```python
from build123d import *

# Parameters (mm, degrees)
F0_W     = 760
F0_H     = 80
F1_DEPTH = 50
F2_W     = 45
F2_H     = 65
F2_W_2   = 50
F2_W_3   = 55
F3_DEPTH = 50


with BuildPart() as f1:
    # F0 (on Front) → F1 (new body)
    with BuildSketch(Plane.XZ):
        with Locations((-24.780855, -40)):
            Rectangle(F0_W, F0_H)
    extrude(amount=F1_DEPTH)

    # F2 (on face) → F3 (cut)
    with BuildSketch(Plane.XZ.offset(50)):
        with Locations((-352.280855, -47.5)):
            Rectangle(F2_W, F2_H)
        with Locations((-274.780855, -47.5)):
            Rectangle(F2_W_2, F2_H)
        with Locations((-192.280855, -47.5)):
            Rectangle(F2_W_3, F2_H)
        with Locations((-107.280855, -47.5)):
            Rectangle(F2_W_3, F2_H)
        with Locations((-24.780855, -47.5)):
            Rectangle(F2_W_2, F2_H)
        with Locations((57.719145, -47.5)):
            Rectangle(F2_W_3, F2_H)
        with Locations((142.719145, -47.5)):
            Rectangle(F2_W_3, F2_H)
        with Locations((225.219145, -47.5)):
            Rectangle(F2_W_2, F2_H)
        with Locations((302.719145, -47.5)):
            Rectangle(F2_W, F2_H)
    extrude(amount=-F3_DEPTH, mode=Mode.SUBTRACT)


solid = f1.part
```
Check sheet for the modelled part. Datum: model origin and axes. Units: mm. A direction names the side the tool comes from. Coordinates: 2 decimals unless noted, no trailing zeros. Write each loop counter-clockwise with the first axis right and the second up, starting at its lowest first coordinate (ties: lowest second). Pieces come first, ordered by that corner, then holes. Notation, with made-up numbers: M 80.25,5.5 L 102.25,5.5 A25 cw 102.25,19.5 Z; hole C -40,-40 d4. An arc over 180 degrees is marked long. Write item = value, one per line. Start each with the question number.
1. Thickness scan on probe 1 along Z at (x, y) = (-215, -30.5). Record the ranges inside material, lowest first.
2. Tool access check on faces 1 (the flat face through (225, -25, -15)), 2 (the flat face through (265, -25, -80)). Record the directions out of +Z, -Z, +X, -X, +Y, -Y that give a thin tool (end or side, any length) a straight path to the whole face; none if there is none.
3. Sectioned sample at B-B (x = -265.5). Record the cut outline in (y, z).
4. Go/stop test with flat-tipped pins: pin 1 (25 mm diameter, centred on x = -99, y = -22.5, fed in from -Z); pin 2 (1 mm diameter, centred on x = -298.5, z = -67.5, fed in from +Y). Record where each tip stops, or that it passes through.
5. Mould release check, pull along X, two halves, no side actions. Record for faces 3 (the flat face through (-404.781, -25, -41)), 4 (the flat face through (115.219, -25, -48)), 5 (the flat face through (15, -25, -80)): pulls with the +X half, pulls with the -X half, needs draft (parallel to the pull), parting line crosses it, or undercut.
6. Sectioned sample at A-A (z = -28.5). State how many separate pieces and enclosed holes the cut face has, then the cut area to 3 significant figures.
The answers:
q1.probe_1 = -15 to 0
q2.face_1 = -Z, +Y, -Y
q2.face_2 = -Z, +X, -X, +Y, -Y
q3.outline = M -50,-15 L 0,-15 L 0,0 L -50,0 Z
q4.pin_1 = -15
q4.pin_2 = through
q5.face_3 = pulls with the -X half
q5.face_4 = undercut
q5.face_5 = needs draft
q6.separate_pieces = 10
q6.enclosed_holes = 0
q6.area = 15,000 mm²
